from build123d import *

# Parameters (mm, degrees)
SKETCH1_R           = 57.5
SKETCH1_R_2         = 1.6
BOSS_EXTRUDE1_DEPTH = 10
FILLET1_R           = 14


with BuildPart() as part:
    # Sketch1 → Boss-Extrude1 (new body)
    with BuildSketch(Plane(origin=(0, 0, 0), x_dir=(1, 0, 0), z_dir=(0, 1, 0))):
        with Locations(Location((0, 0, 0), (0, 0, 270))):
            Circle(SKETCH1_R)
        with Locations(Location((-27, -46.765371804, 0), (0, 0, 270))):
            Circle(SKETCH1_R_2, mode=Mode.SUBTRACT)
        with Locations(Location((-46.765371804, -27, 0), (0, 0, 270))):
            Circle(SKETCH1_R_2, mode=Mode.SUBTRACT)
        with Locations(Location((-54, 0, 0), (0, 0, 270))):
            Circle(SKETCH1_R_2, mode=Mode.SUBTRACT)
        with Locations(Location((0, -54, 0), (0, 0, 270))):
            Circle(SKETCH1_R_2, mode=Mode.SUBTRACT)
        with Locations(Location((27, -46.765371804, 0), (0, 0, 270))):
            Circle(SKETCH1_R_2, mode=Mode.SUBTRACT)
        with Locations(Location((46.765371804, -27, 0), (0, 0, 270))):
            Circle(SKETCH1_R_2, mode=Mode.SUBTRACT)
        with Locations(Location((-46.765371804, 27, 0), (0, 0, 270))):
            Circle(SKETCH1_R_2, mode=Mode.SUBTRACT)
        with Locations(Location((-27, 46.765371804, 0), (0, 0, 270))):
            Circle(SKETCH1_R_2, mode=Mode.SUBTRACT)
        with BuildLine():
            ThreePointArc((43.337291938, 12.119369929), (44.541964885, 6.404167722), (44.996248187, 0.581075772))
            ThreePointArc((44.996248187, 0.581075772), (49.649801174, -1.617727663), (51.541964885, -6.404167722))
            ThreePointArc((51.541964885, -6.404167722), (48.916629323, -11.868809619), (43.009876012, -13.234446171))
            ThreePointArc((43.009876012, -13.234446171), (40.933439791, -18.693675585), (38.167406032, -23.837976356))
            ThreePointArc((38.167406032, -23.837976356), (40.258159872, -26.3152212), (41.008730846, -29.468733028))
            ThreePointArc((41.008730846, -29.468733028), (36.666623102, -35.944503928), (29.027128345, -34.386419122))
            ThreePointArc((29.027128345, -34.386419122), (24.328836786, -37.856408977), (19.22068214, -40.688639423))
            ThreePointArc((19.22068214, -40.688639423), (19.562695248, -41.91207899), (19.677965058, -43.177183813))
            ThreePointArc((19.677965058, -43.177183813), (13.403758509, -50.139455271), (5.828472525, -44.620946965))
            ThreePointArc((5.828472525, -44.620946965), (0, -45), (-5.828472525, -44.620946965))
            ThreePointArc((-5.828472525, -44.620946965), (-14.650092956, -49.893634628), (-19.22068214, -40.688639423))
            ThreePointArc((-19.22068214, -40.688639423), (-24.328836785, -37.856408977), (-29.027128345, -34.386419122))
            ThreePointArc((-29.027128345, -34.386419122), (-39.298977866, -34.052758165), (-38.167406032, -23.837976356))
            ThreePointArc((-38.167406032, -23.837976356), (-40.933439791, -18.693675585), (-43.009876012, -13.234446171))
            ThreePointArc((-43.009876012, -13.234446171), (-51.470714978, -7.40037159), (-44.996248187, 0.581075772))
            ThreePointArc((-44.996248187, 0.581075772), (-44.541964885, 6.404167722), (-43.337291938, 12.119369929))
            ThreePointArc((-43.337291938, 12.119369929), (-47.300863758, 21.601580676), (-37.539099471, 24.815640449))
            ThreePointArc((-37.539099471, 24.815640449), (-34.008730846, 29.468733028), (-29.905423881, 33.625371708))
            ThreePointArc((-29.905423881, 33.625371708), (-28.113322508, 43.745183707), (-18.163551911, 41.171414622))
            ThreePointArc((-18.163551911, 41.171414622), (-12.677965058, 43.177183813), (-6.978795043, 44.455555556))
            ThreePointArc((-6.978795043, 44.455555556), (-0.272428616, 51.994696752), (7, 45))
            ThreePointArc((7, 45), (6.994696752, 44.727571384), (6.978795043, 44.455555556))
            ThreePointArc((6.978795043, 44.455555556), (12.677965058, 43.177183813), (18.163551911, 41.171414622))
            ThreePointArc((18.163551911, 41.171414622), (26.038077243, 44.644523374), (31.328836786, 37.856408977))
            ThreePointArc((31.328836786, 37.856408977), (30.963447161, 35.624381834), (29.905423881, 33.625371708))
            ThreePointArc((29.905423881, 33.625371708), (34.008730846, 29.468733028), (37.539099471, 24.815640449))
            ThreePointArc((37.539099471, 24.815640449), (44.485876825, 24.725274968), (47.933439791, 18.693675585))
            ThreePointArc((47.933439791, 18.693675585), (46.670467115, 14.68287548), (43.337291938, 12.119369929))
        make_face(mode=Mode.SUBTRACT)
        with Locations(Location((54, 0, 0), (0, 0, 270))):
            Circle(SKETCH1_R_2, mode=Mode.SUBTRACT)
        with Locations(Location((46.765371804, 27, 0), (0, 0, 270))):
            Circle(SKETCH1_R_2, mode=Mode.SUBTRACT)
        with Locations(Location((0, 54, 0), (0, 0, 270))):
            Circle(SKETCH1_R_2, mode=Mode.SUBTRACT)
        with Locations(Location((27, 46.765371804, 0), (0, 0, 270))):
            Circle(SKETCH1_R_2, mode=Mode.SUBTRACT)
    extrude(amount=BOSS_EXTRUDE1_DEPTH)

    # Fillet1
    # the kernel refuses this fillet: 14 mm, written as the material it takes off along each edge
    with BuildSketch(Plane(origin=(43.009876012, -16.77410228, 13.234446171), x_dir=(-0.3645348982341331, 0, 0.9311897271605987), z_dir=(0, 1, 0)), Plane(origin=(43.337291938, -16.77410228, -12.119369929), x_dir=(0.19677290431862063, 0, 0.9804490930823564), z_dir=(0, 1, 0)), Plane(origin=(29.027128345, -16.77410228, 34.386419122), x_dir=(-0.8101054462780665, 0, 0.586284202337582), z_dir=(0, 1, 0)), Plane(origin=(5.828472525, -16.77410228, 44.620946965), x_dir=(-0.9984732390602963, 0, 0.05523758575861507), z_dir=(0, 1, 0)), Plane(origin=(-19.22068214, -16.77410228, 40.688639423), x_dir=(-0.8698328333156817, 0, -0.4933465740085904), z_dir=(0, 1, 0)), Plane(origin=(-38.167406032, -16.77410228, 23.837976356), x_dir=(-0.46502664893844664, 0, -0.8852966823483972), z_dir=(0, 1, 0)), Plane(origin=(-44.996248187, -16.77410228, -0.581075772), x_dir=(0.0874222107554752, 0, -0.99617134925003), z_dir=(0, 1, 0)), Plane(origin=(-37.539099471, -16.77410228, -24.815640449), x_dir=(0.6121151362303556, 0, -0.7907686513751624), z_dir=(0, 1, 0)), Plane(origin=(-18.163551911, -16.77410228, -41.171414622), x_dir=(0.9424658309509625, 0, -0.334302493992958), z_dir=(0, 1, 0)), Plane(origin=(6.978795043, -16.77410228, -44.455555556), x_dir=(0.9735902834899675, 0, 0.22830234316345693), z_dir=(0, 1, 0))) as fillet1_piece_1:
        with BuildLine():
            CenterArc((7.753362832, 13.961040239), FILLET1_R, 225.679308165, 40.045235058)
            ThreePointArc((-2.028069047, 3.944873787), (-0.693306264, 2.137324059), (0, 0))
            ThreePointArc((0, 0), (3.354820456, 0.125227803), (6.709640912, 0))
        make_face()
    extrude(amount=43.54820456, mode=Mode.SUBTRACT)
    with BuildSketch(Plane(origin=(44.996248187, -16.77410228, -0.581075772), x_dir=(0.9259201789863998, 0, 0.37771923719317424), z_dir=(0, 1, 0)), Plane(origin=(37.539099471, -16.77410228, -24.815640449), x_dir=(0.9831440588568181, 0, -0.18283259975874497), z_dir=(0, 1, 0)), Plane(origin=(38.167406032, -16.77410228, 23.837976356), x_dir=(0.5747231845271455, 0, 0.8183478851729116), z_dir=(0, 1, 0)), Plane(origin=(19.22068214, -16.77410228, 40.688639423), x_dir=(0.041055639780420296, 0, 0.9991568617800813), z_dir=(0, 1, 0)), Plane(origin=(-5.828472525, -16.77410228, 44.620946965), x_dir=(-0.5056467805113274, 0, 0.8627405944770012), z_dir=(0, 1, 0)), Plane(origin=(-29.027128345, -16.77410228, 34.386419122), x_dir=(-0.8918099207200904, 0, 0.4524102842611189), z_dir=(0, 1, 0)), Plane(origin=(-43.009876012, -16.77410228, 13.234446171), x_dir=(-0.994829712327915, 0, -0.10155709462936494), z_dir=(0, 1, 0)), Plane(origin=(-43.337291938, -16.77410228, -12.119369929), x_dir=(-0.7819980994024467, 0, -0.62328081354311), z_dir=(0, 1, 0)), Plane(origin=(-29.905423881, -16.77410228, -33.625371708), x_dir=(-0.3208876152512941, 0, -0.9471172780486783), z_dir=(0, 1, 0)), Plane(origin=(18.163551911, -16.77410228, -41.171414622), x_dir=(0.7282266466043301, 0, -0.6853363781205636), z_dir=(0, 1, 0)), Plane(origin=(-6.978795043, -16.77410228, -44.455555556), x_dir=(0.24210241945853378, 0, -0.9702506987847646), z_dir=(0, 1, 0))) as fillet1_piece_2:
        with BuildLine():
            CenterArc((8.87132307, 13.278738899), FILLET1_R, 211.483261097, 40.045235058)
            ThreePointArc((-3.067775786, 5.967246676), (-1.422516032, 3.040879878), (0, 0))
            ThreePointArc((0, 0), (2.217830767, 0.36063055), (4.435661535, 0))
        make_face()
    extrude(amount=43.54820456, mode=Mode.SUBTRACT)
    with BuildSketch(Plane(origin=(29.905423881, -16.77410228, -33.625371708), x_dir=(0.3208876152513925, 0, -0.9471172780486449), z_dir=(0, 1, 0))) as fillet1_piece_3:
        with BuildLine():
            CenterArc((8.87132307, -13.278738899), FILLET1_R, 108.471503845, 40.045235058)
            ThreePointArc((-3.067775786, -5.967246676), (-1.422516032, -3.040879878), (0, 0))
            ThreePointArc((0, 0), (2.217830767, -0.36063055), (4.435661535, 0))
        make_face()
    extrude(amount=43.54820456, mode=Mode.SUBTRACT)


solid = part.part
The model under review builds one solid part; all positions refer to its coordinate system, in mm. A direction names the side the tool comes from. Coordinates: 2 decimals unless noted, no trailing zeros. Order: outer loops, then holes, each group sorted by start corner. A loop starts at its lowest first (then second) coordinate and runs counter-clockwise, first axis right, second up. Notation, with made-up numbers: (44, -14) -> (53, -14) arc R19 ccw to (53, 17) -> close; hole circle Ø8 at (-12, 10). An arc over 180 degrees is marked (long way). Answer in a Markdown table with one row per item.
(1) The part is to be moulded in two halves that separate along Z. For faces 1 (the flat face through (-25, 0, 38)), 2 (the cylindrical face through (37.602, 4.93, -26.956)), say which applies: +Z half, -Z half, draft (parallel to the pull), parting line (faces both ways), or undercut.
Answers:
| item | result |
|---|---|
| face 1 | draft |
| face 2 | undercut |
(2) Consider section C-C (y = 2). State how many separate pieces and enclosed holes the cut face has, plus the area to 3 significant figures.
Answers:
| item | result |
|---|---|
| separate pieces | 1 |
| enclosed holes | 13 |
| area | 2,920 mm² |
(3) Insertion check: pin 1 (3 mm diameter, centred on y = 4.5, z = 5, fed in from -X); pin 2 (1.5 mm diameter, centred on x = -30.5, y = 2, fed in from +Z); pin 3 (5 mm diameter, centred on x = 27, z = 46.77, fed in from +Y); pin 4 (4 mm diameter, centred on y = 1, z = 26.5, fed in from -X). Each pin has a flat end and moves straight along its axis. Give the tip position at first contact, or say it passes through.
Answers:
| item | result |
|---|---|
| pin 1 | x = -57.39 |
| pin 2 | z = 49.21 |
| pin 3 | y = 10 |
| pin 4 | x = -52.02 |
(4) Machinability: for faces 3 (the cylindrical face through (-4.25, 4.93, 46.07)), 4 (the flat face through (-25, 10, 38)), which of the approach directions +Z, -Z, +X, -X, +Y, -Y give a long, thin tool a straight path to every point of the face, cutting with its end or side? Answer none if there is none.
Answers:
| item | result |
|---|---|
| face 3 | +Y, -Y |
| face 4 | +Z, -Z, +X, -X, +Y |
(5) Wall thickness on line 1 along X through (y, z) = (4, 0); line 2 along X through (y, z) = (4, -28); line 3 along X through (y, z) = (6, 49): over which ranges is each line inside the solid? List them lowest first.
Answers:
| item | result |
|---|---|
| line 1 | -57.5 to -55.6, -52.4 to -47.97, 47.97 to 52.4, 55.6 to 57.5 |
| line 2 | -50.22 to -48.01, -45.52 to -35.84, 35.84 to 45.52, 48.01 to 50.22 |
| line 3 | -30.09 to -16.56, -8.79 to 8.79, 16.56 to 30.09 |
(6) Consider section A-A (x = -36). Write out the cut boundary in (y, z).
Answers:
| item | result |
|---|---|
| outline | (0, -44.84) -> (10, -44.84) -> (10, -27.89) -> (0, -27.89) -> close; (0, 36.18) -> (10, 36.18) -> (10, 44.84) -> (0, 44.84) -> close |
(7) Consider section B-B (z = -35.5). Write out the cut boundary in (x, y), plus the area to 3 significant figures.
Answers:
| item | result |
|---|---|
| outline | (-45.23, 0) -> (-31.51, 0) -> (-31.51, 10) -> (-45.23, 10) -> close; (31.51, 0) -> (45.23, 0) -> (45.23, 10) -> (31.51, 10) -> close |
| area | 274 mm² |
